The listing builds one solid part. Answer for the finished solid, in the listing's coordinates (mm). Face numbers are marked on the shaded views. Round coordinates to 2 decimals unless told otherwise and drop trailing zeros. Write each loop counter-clockwise with the first axis right and the second up, starting at its lowest first coordinate (ties: lowest second). Pieces come first, ordered by that corner, then holes. Notation, with made-up numbers: (89.25, -37.75) -> (141.25, -37.75) arc R21 ccw to (141.25, -9.75) -> close; hole circle Ø4 at (20.25, -7.75). An arc over 180 degrees is marked (long way). Write each question's results on one line, items separated by ' | '. Start each with the question number.
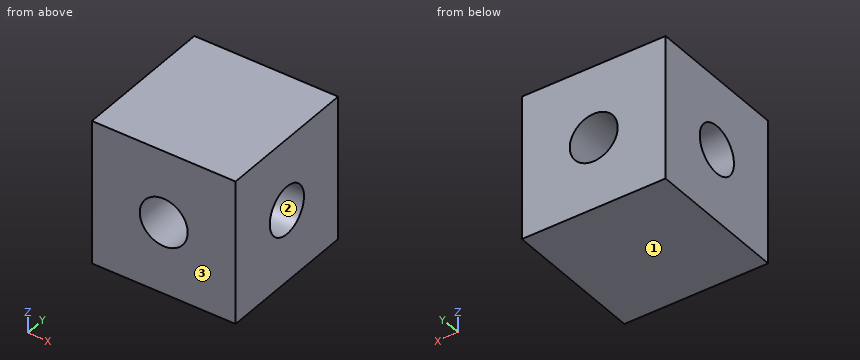
```python
from build123d import *

# Parameters (mm, degrees)
F0_W       = 38.1
F0_H       = 38.1
F1_DEPTH   = 19.05
F4_D       = 12.7
F4_ON_F3_D = 12.7


with BuildPart() as f1:
    # F0 (on Front) → F1 (new body, symmetric)
    with BuildSketch(Plane.XZ):
        Rectangle(F0_W, F0_H)
    extrude(amount=F1_DEPTH, both=True)

    # F4 (through all)
    with Locations(Plane.XZ.offset(19.05)):
        with Locations((0, 0)):
            Hole(F4_D / 2)

    # F4 on F3 (through all)
    with Locations(Plane(origin=(-19.05, 0, 0), x_dir=(0, -1, 0), z_dir=(-1, 0, 0))):
        with Locations((0, 0)):
            Hole(F4_ON_F3_D / 2)


solid = f1.part
```
Q1. The part is cut by section A-A, the plane y = 4. Write down the section's boundary in (x, z), then the cut area to 3 significant figures.
Q2. The part is cut by section D-D, the plane x = -3. Write down the section's boundary in (y, z).
Q3. The part is cut by section B-B, the plane z = 0. Write down the section's boundary in (x, y), then the cut area to 3 significant figures.
Q4. Each of these flat-tipped pins is pushed along its axis until it touches: pin 1 (20.5 mm diameter, centred on x = 0, z = 0, fed in from +Y); pin 2 (10 mm diameter, centred on y = 0, z = 0, fed in from -X). Where does it stop, or does it pass through?
Q5. Find the intervals of material crossed by line 1 (X direction, y = 10, z = 0); line 2 (Y direction, x = -10, z = -4.5), in increasing order.
Q6. The part is cut by section C-C, the plane x = 15. Write down the section's boundary in (y, z), then the cut area to 3 significant figures.
Q7. Determine the mould class of the marked faces 1, 2 and 3 for opening direction Z: pulls with the +Z half, pulls with the -Z half, needs draft (parallel to the pull), parting line crosses it, or undercut.
Answers follow:
1) outline: (-19.05, -19.05) -> (19.05, -19.05) -> (19.05, -4.93) -> (4, -4.93) arc R6.35 cw to (-4, -4.93) -> (-19.05, -4.93) -> close; (-19.05, 4.93) -> (-4, 4.93) arc R6.35 cw to (4, 4.93) -> (19.05, 4.93) -> (19.05, 19.05) -> (-19.05, 19.05) -> close | area: 1,060 mm^2
2) outline: (-19.05, -19.05) -> (19.05, -19.05) -> (19.05, -5.6) -> (3, -5.6) arc R6.35 cw to (-3, -5.6) -> (-19.05, -5.6) -> close; (-19.05, 5.6) -> (-3, 5.6) arc R6.35 cw to (3, 5.6) -> (19.05, 5.6) -> (19.05, 19.05) -> (-19.05, 19.05) -> close
3) outline: (-19.05, -19.05) -> (-6.35, -19.05) -> (-6.35, -6.35) -> (-19.05, -6.35) -> close; (-19.05, 6.35) -> (-6.35, 6.35) -> (-6.35, 19.05) -> (-19.05, 19.05) -> close; (6.35, -19.05) -> (19.05, -19.05) -> (19.05, -6.35) -> (6.35, -6.35) -> close; (6.35, 6.35) -> (19.05, 6.35) -> (19.05, 19.05) -> (6.35, 19.05) -> close | area: 645 mm^2
4) pin 1: y = 19.05 | pin 2: through
5) line 1: -19.05 to -6.35, 6.35 to 19.05 | line 2: -19.05 to -4.48, 4.48 to 19.05
6) outline: (-19.05, -19.05) -> (19.05, -19.05) -> (19.05, 19.05) -> (-19.05, 19.05) -> close; hole circle Ø12.7 at (0, 0) | area: 1,320 mm^2
7) face 1: pulls with the -Z half | face 2: undercut | face 3: needs draft
